from build123d import *

# Parameters (mm, degrees)
SKETCH1_R           = 1
BOSS_EXTRUDE1_DEPTH = 20
SKETCH2_R           = 1.7
CUT_EXTRUDE1_DEPTH  = 33.496153619
SKETCH3_W           = 20
SKETCH3_H           = 4
CUT_EXTRUDE2_DEPTH  = 33.496153619
CUT_EXTRUDE3_DEPTH  = 28.730849248
FILLET1_DEPTH       = 20
FILLET1_2_DEPTH     = 5
FILLET1_START       = 15
FILLET1_3_DEPTH     = 5
FILLET2_R           = 1


with BuildPart() as part:
    # Sketch1 → Boss-Extrude1 (new body)
    with BuildSketch(Plane.XY):
        with BuildLine():
            Line((5, 0), (5, 5))
            Line((5, 5), (10, 5))
            Line((10, 5), (10, 16))
            Line((10, 16), (-10, 16))
            Line((-10, 16), (-10, 5))
            Line((-10, 5), (-5, 5))
            Line((-5, 5), (-5, 0))
            ThreePointArc((-5, 0), (0, -5), (5, 0))
        make_face()
        Circle(SKETCH1_R, mode=Mode.SUBTRACT)
    extrude(amount=BOSS_EXTRUDE1_DEPTH)

    # Sketch2 → Cut-Extrude1 (cut, through all)
    with BuildSketch(Plane(origin=(10, 0, 0), x_dir=(0, 0, -1), z_dir=(1, 0, 0))):
        with Locations((-17, 8)):
            Circle(SKETCH2_R)
        with Locations(Location((-3, 8, 0), (0, 0, 180))):
            Circle(SKETCH2_R)
    extrude(amount=-CUT_EXTRUDE1_DEPTH, mode=Mode.SUBTRACT)

    # Sketch3 → Cut-Extrude2 (cut, through all)
    with BuildSketch(Plane(origin=(10, 0, 0), x_dir=(0, 0, -1), z_dir=(1, 0, 0))):
        with Locations((-10, 14)):
            Rectangle(SKETCH3_W, SKETCH3_H)
    extrude(amount=-CUT_EXTRUDE2_DEPTH, mode=Mode.SUBTRACT)

    # Sketch4 → Cut-Extrude3 (cut, through all)
    with BuildSketch(Plane(origin=(5, 0, 0), x_dir=(0, 0, -1), z_dir=(1, 0, 0))):
        Polygon((-10, -5), (-15, -5), (-15, 2), (-5, 2), (-5, -5), align=None)
    extrude(amount=-CUT_EXTRUDE3_DEPTH, mode=Mode.SUBTRACT)

    # Fillet1: read off the stored shape, not the designer's step
    # Fillet1 outline → Fillet1 (add)
    with BuildSketch(Plane.XY):
        with BuildLine():
            Line((5, 2), (6.4306416, 2))
            ThreePointArc((6.4306416, 2), (8.038028722, 3.710939656), (10, 5))
            Line((10, 5), (5, 5))
            Line((5, 5), (5, 2))
        make_face()
        with BuildLine():
            Line((-6.4306416, 2), (-5, 2))
            Line((-5, 2), (-5, 5))
            Line((-5, 5), (-10, 5))
            ThreePointArc((-10, 5), (-8.038028722, 3.710939656), (-6.4306416, 2))
        make_face()
    extrude(amount=FILLET1_DEPTH)

    # Fillet1 2 outline → Fillet1 2 (add)
    with BuildSketch(Plane.XY):
        with BuildLine():
            ThreePointArc((4.824045318, -1.314757303), (5.473399472, 0.417234907), (6.4306416, 2))
            Line((6.4306416, 2), (5, 2))
            Line((5, 2), (5, 0))
            ThreePointArc((5, 0), (4.955816204, -0.663238839), (4.824045318, -1.314757303))
        make_face()
        with BuildLine():
            Line((-5, 0), (-5, 2))
            Line((-5, 2), (-6.4306416, 2))
            ThreePointArc((-6.4306416, 2), (-5.473399472, 0.417234907), (-4.824045318, -1.314757303))
            ThreePointArc((-4.824045318, -1.314757303), (-4.955816204, -0.663238839), (-5, 0))
        make_face()
    extrude(amount=FILLET1_2_DEPTH)

    # Fillet1 3 outline → Fillet1 3 (add)
    with BuildSketch(Plane.XY.offset(FILLET1_START)):
        with BuildLine():
            ThreePointArc((4.824045318, -1.314757303), (5.473399472, 0.417234907), (6.4306416, 2))
            Line((6.4306416, 2), (5, 2))
            Line((5, 2), (5, 0))
            ThreePointArc((5, 0), (4.955816204, -0.663238839), (4.824045318, -1.314757303))
        make_face()
        with BuildLine():
            Line((-5, 0), (-5, 2))
            Line((-5, 2), (-6.4306416, 2))
            ThreePointArc((-6.4306416, 2), (-5.473399472, 0.417234907), (-4.824045318, -1.314757303))
            ThreePointArc((-4.824045318, -1.314757303), (-4.955816204, -0.663238839), (-5, 0))
        make_face()
    extrude(amount=FILLET1_3_DEPTH)

    # Fillet2
    fillet2_edges = [part.edges().sort_by_distance(p)[0] for p in [
        (10, 8.5, 0),
        (-10, 5, 10),
        (10, 5, 10),
        (10, 8.5, 20),
        (-10, 8.5, 0),
        (-10, 8.5, 20),
        (-10, 12, 10),
        (0, 12, 0),
        (0, 12, 20),
        (10, 12, 10),
        (0, -5, 0),
        (0, -5, 20),
        (8.038028722, 3.710939656, 0),
        (8.038028722, 3.710939656, 20),
        (-8.038028722, 3.710939656, 0),
        (-8.038028722, 3.710939656, 20),
    ]]
    fillet(fillet2_edges, radius=FILLET2_R)


solid = part.part
Input: part model. Units: mm. Frame: model coordinates. A direction names the side the tool comes from. Give positions to 0.01 mm unless a question says otherwise; leave off trailing zeros. Write each loop counter-clockwise with the first axis right and the second up, starting at its lowest first coordinate (ties: lowest second). Pieces come first, ordered by that corner, then holes.
Q1. Section B-B, the plane x = 0. Output: boundary loops of the cut face in (y, z).
Q2. Section D-D, the plane z = 6. Output: boundary loops of the cut face in (x, y).
Q3. Pull-direction query (X, two-part tool) for faces 3 (the face through (0, 12, 10)), 4 (the face through (-9.86, 5.09, 10.13)), 5 (the face through (0, -1, 2)); classes: pulls with the +X half, pulls with the -X half, needs draft (parallel to the pull), parting line crosses it, or undercut.
Q4. Material intervals for probe 1 along Z at (x, y) = (2.25, 7.5); probe 2 along Y at (x, z) = (2.5, 10); probe 3 along Z at (x, y) = (-3.75, 9), sorted ascending.
Q5. Section A-A, the plane z = 17. Output: boundary loops of the cut face in (x, y), plus the area to 3 significant figures.
Q6. Set-up query: faces 1 (the face through (-0.1, -1.5, 15)), 2 (the face through (0.14, 8.51, 15.38)). Return all of +Z, -Z, +X, -X, +Y, -Y with unobstructed straight access to the full face (end or side cutting, diameter ignored); none if empty.
Q7. Section C-C, the plane y = 8. Output: boundary loops of the cut face in (x, z), plus the area to 3 significant figures.
Q8. First-contact query: P1, Ø4, axis at y = 3.5, z = 16, coming from the +X side. Flat tip, straight axial feed; report the tip coordinate or a pass-through.
Filled in:
1. outline: (-5, 1) arc R1 ccw to (-4, 0) - (-1, 0) - (-1, 5) - (-5, 5) - close; (-5, 15) - (-1, 15) - (-1, 20) - (-4, 20) arc R1 ccw to (-5, 19) - close; (1, 0) - (11, 0) arc R1 ccw to (12, 1) - (12, 19) arc R1 ccw to (11, 20) - (1, 20) - (1, 15) - (2, 15) - (2, 5) - (1, 5) - close; hole circle Ø3.4 at (8, 3); hole circle Ø3.4 at (8, 17)
2. outline: (-10, 5.6) arc R1 ccw to (-9.5, 4.73) arc R10 cw to (-6.43, 2) - (6.43, 2) arc R10 cw to (9.5, 4.73) arc R1 ccw to (10, 5.6) - (10, 11) arc R1 ccw to (9, 12) - (-9, 12) arc R1 ccw to (-10, 11) - close
3. face 3: needs draft
3. face 4: pulls with the -X half
3. face 5: undercut
4. probe 1: z = 0 to 1.38, 4.62 to 15.38, 18.62 to 20
4. probe 2: y = 2 to 12
4. probe 3: z = 0 to 1.63, 4.37 to 15.63, 18.37 to 20
5. outline: (-10, 5.6) arc R1 ccw to (-9.5, 4.73) arc R10 cw to (-4.82, -1.31) arc R5 ccw to (4.82, -1.31) arc R10 cw to (9.5, 4.73) arc R1 ccw to (10, 5.6) - (10, 6.3) - (-10, 6.3) - close; (-10, 9.7) - (10, 9.7) - (10, 11) arc R1 ccw to (9, 12) - (-9, 12) arc R1 ccw to (-10, 11) - close; hole circle Ø2 at (0, 0)
5. area: 179 mm2
6. face 1: +X, -X, -Y
6. face 2: +X, -X
7. outline: (-10, 1) arc R1 ccw to (-9, 0) - (9, 0) arc R1 ccw to (10, 1) - (10, 1.3) - (-10, 1.3) - close; (-10, 4.7) - (10, 4.7) - (10, 15.3) - (-10, 15.3) - close; (-10, 18.7) - (10, 18.7) - (10, 19) arc R1 ccw to (9, 20) - (-9, 20) arc R1 ccw to (-10, 19) - close
7. area: 263 mm2
8. P1: stops at x = 10
